Can you work these out from the model? Positions are in its coordinate system, mm. Give positions to 0.01 mm unless a question says otherwise; leave off trailing zeros. Order: outer loops, then holes, each group sorted by start corner. A loop starts at its lowest first (then second) coordinate and runs counter-clockwise, first axis right, second up. Notation, with made-up numbers: (33, 26) - (62, 26) arc R21 cw to (62, 51) - close; hole circle Ø10 at (-8.5, -21.75). An arc over 180 degrees is marked (long way). Answer as CSV lines item,"result".
Autodesk Inventor part; units mm, degrees
ref_plane "YZ Plane" through (0, 0, 0) normal (1, 0, 0) x (0, 1, 0)
ref_plane "XZ Plane" through (0, 0, 0) normal (0, 1, 0) x (-1, 0, 0)
ref_plane "XY Plane" through (0, 0, 0) normal (0, 0, 1) x (1, 0, 0)
sketch "Sketch1" plane through (0, 0, 0) normal (0, 1, 0) x (-1, 0, 0)
  arc A0 (5.45, 0) -> (-3.8537, 3.8537) centre (0, 0) ccw
  line L0 (5.45, 0) -> (5.45, -170)
  line L1 (-3.8537, 3.8537) -> (-14.7075, -7)
  arc A1 (-14.7075, -7) -> (-16.7785, -12) centre (-9.7075, -12) ccw
  line L2 (-16.7785, -12) -> (-16.7785, -158)
  arc A2 (-3.8537, -173.8537) -> (5.45, -170) centre (0, -170) ccw
  line L3 (-3.8537, -173.8537) -> (-14.7075, -163)
  arc A3 (-16.7785, -158) -> (-14.7075, -163) centre (-9.7075, -158) ccw
  dimension "d0" = 10.9
  dimension "d3" = 170
  dimension "d5" = 0
  dimension "d6" = 12
  dimension "d7" = 12
  dimension "d8" = 5.45
  dimension "d9" = 45
  dimension "d10" = 7
  dimension "d11" = 7
  dimension "d12" = 10.9
  dimension "d13" = 135
extrude "Extrusion1" add sketch "Sketch1" along normal blind 1.7
sketch "Sketch2" plane through (0, 1.7, 0) normal (0, 1, 0) x (1, 0, 0)
  arc A0 (3.8537, 173.8537) -> (-5.45, 170) centre (0, 170) ccw
  arc A1 (-5.45, 0) -> (3.8537, -3.8537) centre (0, 0) ccw
  circle A2 centre (0, 0) radius 1.5
  circle A3 centre (0, 170) radius 1.5
  dimension "d16" = 3
  dimension "d17" = 3
extrude "Extrusion2" cut sketch "Sketch2" against normal blind 1.7
equation "\"BendRadius\" = Thickness"
equation "\"BendReliefWidth\" = Thickness"
equation "\"BendReliefDepth\" = 0.5 * Thickness"
equation "\"CornerReliefSize\" = 4 * Thickness"
equation "\"MinimumRemnant\" = 2 * Thickness"
equation "\"TransitionRadius\" = BendRadius"
equation "\"JacobiRadiusSize\" = BendRadius"
equation "\"GapSize\" = Thickness"
properties part number "A3P2"
1) I'm going to push flat-ended pins straight in: P1, Ø1, axis at x = -2.5, y = 1.5, coming from the +Z side; P2, Ø1.8, axis at x = 0, z = 0, coming from the -Y side. Where does each tip first touch, or does it pass through?
Answer block:
P1,"z = 5.07"
P2,"through"
2) If we mould it in two halves opening along X, with no side actions, what happens to faces 1 (the flat face through (9.205, 0.838, -1.497)), 2 (the cylindrical face through (-0.195, 0.862, -171.487)), 3 (the cylindrical face through (-2.17, 0.84, -175)), 4 (the cylindrical face through (-1.5, 0.86, -0.07))? For each: +X half, -X half, draft (parallel to the pull), parting line (faces both ways), or undercut.
Answer block:
face 1,"+X half"
face 2,"undercut"
face 3,"parting line"
face 4,"undercut"
3) I want a section at B-B on y = 1.25. Write out the boundary of the cut face in (x, z), plus the area to 3 significant figures.
Answer block:
outline,"(-5.45, -170) arc R5.45 ccw to (3.85, -173.85) - (14.71, -163) arc R7.07 ccw to (16.78, -158) - (16.78, -12) arc R7.07 ccw to (14.71, -7) - (3.85, 3.85) arc R5.45 ccw to (-5.45, 0) - close; hole circle Ø3 at (0, -170); hole circle Ø3 at (0, 0)"
area,"3,780 mm2"
4) I want a section at C-C on x = 7.25. Write out the boundary of the cut face in (y, z), plus the area to 3 significant figures.
Answer block:
outline,"(0, -170.46) - (1.7, -170.46) - (1.7, 0.46) - (0, 0.46) - close"
area,"291 mm2"
5) I want a section at A-A on x = 0. Write out the boundary of the cut face in (y, z), plus the area to 3 significant figures.
Answer block:
outline,"(0, -175.45) - (1.7, -175.45) - (1.7, -171.5) - (0, -171.5) - close; (0, -168.5) - (1.7, -168.5) - (1.7, -1.5) - (0, -1.5) - close; (0, 1.5) - (1.7, 1.5) - (1.7, 5.45) - (0, 5.45) - close"
area,"297 mm2"
6) I need wall thicknesses on line 1 along Z through (x, y) = (0, 0.9); line 2 along Z through (x, y) = (-1, 0.2); line 3 along X through (y, z) = (0.9, -170). Which ranges of each line are inside material? Lowest first, please. Write a range as [from, to].
Answer block:
line 1,"[-175.45, -171.5], [-168.5, -1.5], [1.5, 5.45]"
line 2,"[-175.36, -171.12], [-168.88, -1.12], [1.12, 5.36]"
line 3,"[-5.45, -1.5], [1.5, 7.71]"
